Here's how the part is built. I have some questions about the finished solid (model axes, mm). Face numbers are marked on the shaded views. A direction names the side the tool comes from. Coordinates: 2 decimals unless noted, no trailing zeros. Loops run counter-clockwise (first coordinate to the right, second up) from the corner with the lowest first, then second, coordinate; pieces in that order, holes last. Notation, with made-up numbers: (-30.75, 3.5) -> (-1.75, 3.5) arc R12 cw to (-1.75, 17.5) -> close; hole circle Ø7 at (-16.5, 40.5). An arc over 180 degrees is marked (long way). Answer as a JSON object with one key per item and string values. Group by question number.
1) Which directions (+Z, -Z, +X, -X, +Y, -Y) give clear straight access to the entire face, cutting with the end or side of a thin tool? Please do the marked faces 1, 2, 3, 4 and 5.
2) I want a section at D-D (x = 11.5). Write out the boundary of the cut face in (y, z).
3) I want a section at A-A (y = 0). Write out the boundary of the cut face in (x, z) (3 decimals).
4) I want a section at C-C (x = 0). Count the separate pieces of the cut face and the enclosed holes in it, then the cut area to 3 significant figures.
5) If we mould it in two halves opening along X, with no side actions, what happens to the marked faces 6, 7, 8 and 9? For each: +X half, -X half, draft (parallel to the pull), parting line (faces both ways), or undercut.
6) I need wall thicknesses on probe 1 along Y at (x, z) = (0, 10) (3 decimals); probe 2 along Y at (x, z) = (0, 12); probe 3 along Z at (x, y) = (5, 19.5). Which ranges of each line are inside material? Lowest first, please. Write a range as [from, to].
7) I'm going to push flat-ended pins straight in: pin 1 (14 mm diameter, centred on x = -4, y = -5.5, fed in from -Z); pin 2 (3.5 mm diameter, centred on x = 0, z = 14, fed in from +Y); pin 3 (3 mm diameter, centred on y = 2, z = 5, fed in from -X); pin 4 (3 mm diameter, centred on x = -12.5, y = 12, fed in from -Z). Where does each tip first touch, or does it pass through?
8) I want a section at B-B (z = 6.75). Write out the boundary of the cut face in (x, y), then the cut area to 4 significant figures.
```python
from build123d import *
from build123d.topology import SkipClean

# Parameters (mm, degrees)
SKETCH2_R           = 14
SKETCH2_R_2         = 3.5
BOSS_EXTRUDE1_DEPTH = 5.5
SKETCH3_R           = 7
CUT_EXTRUDE1_DEPTH  = 39.255719
TAP1_REACH          = 49.937
TAP1_BORE_R         = 1.3105
CIRPATTERN1_COUNT   = 2
CIRPATTERN1_ANGLE   = 120


with BuildPart() as part:
    # Sketch1 → Revolve1 (revolve)
    with BuildSketch(Plane(origin=(0, 0, 0), x_dir=(0, 0, -1), z_dir=(1, 0, 0)), mode=Mode.PRIVATE) as revolve1_sk:
        with BuildLine():
            Line((-11.5, 19), (0, 19))
            Line((0, 19), (0, 14))
            Line((0, 14), (-1.5, 14))
            Line((-1.5, 14), (-1.5, 8.425))
            ThreePointArc((-1.5, 8.425), (-1.55, 8.375), (-1.5, 8.325))
            Line((-1.5, 8.325), (-1.5, 6))
            Line((-1.5, 6), (-16, 6))
            Line((-16, 6), (-16, 9.5))
            Line((-16, 9.5), (-11.5, 9.5))
            Line((-11.5, 9.5), (-11.5, 8.375))
            Line((-11.5, 8.375), (-9.5, 8.375))
            Line((-9.5, 8.375), (-9.5, 14))
            Line((-9.5, 14), (-11.5, 14))
            Line((-11.5, 14), (-11.5, 19))
        make_face()
    revolve(revolve1_sk.sketch.rotate(Axis((0, 0, 16), (0, 0, -1)), 90), axis=Axis((0, 0, 16), (0, 0, -1)))

    # Sketch2 → Boss-Extrude1 (add)
    with SkipClean():  # the faces are left unmerged after this step: merging them gives an invalid solid
        with BuildSketch(Plane.XY):
            with BuildLine():
                Line((-5.76484, 29.278248), (-12.6665, 14.161913))
                ThreePointArc((-12.6665, 14.161913), (-19, 0), (-12.6665, -14.161913))
                Line((-12.6665, -14.161913), (-5.76484, -29.278248))
                ThreePointArc((-5.76484, -29.278248), (-4.850203, -30.524474), (-3.514877, -31.303285))
                ThreePointArc((-3.514877, -31.303285), (0, -31.5), (3.514877, -31.303285))
                ThreePointArc((3.514877, -31.303285), (4.850203, -30.524474), (5.76484, -29.278248))
                Line((5.76484, -29.278248), (12.6665, -14.161913))
                ThreePointArc((12.6665, -14.161913), (19, 0), (12.6665, 14.161913))
                Line((12.6665, 14.161913), (5.76484, 29.278248))
                ThreePointArc((5.76484, 29.278248), (4.850203, 30.524474), (3.514877, 31.303285))
                ThreePointArc((3.514877, 31.303285), (0, 31.5), (-3.514877, 31.303285))
                ThreePointArc((-3.514877, 31.303285), (-4.850203, 30.524474), (-5.76484, 29.278248))
            make_face()
            Circle(SKETCH2_R, mode=Mode.SUBTRACT)
            with Locations((0, 24)):
                Circle(SKETCH2_R_2, mode=Mode.SUBTRACT)
            with Locations((0, -24)):
                Circle(SKETCH2_R_2, mode=Mode.SUBTRACT)
        extrude(amount=BOSS_EXTRUDE1_DEPTH)

    # Sketch3 → Cut-Extrude1 (cut, through all)
    with SkipClean():  # the faces are left unmerged after this step: merging them gives an invalid solid
        with BuildSketch(Plane.XY.offset(5.5)):
            with Locations((0, 24)):
                Circle(SKETCH3_R)
            with Locations((0, -24)):
                Circle(SKETCH3_R)
        extrude(amount=CUT_EXTRUDE1_DEPTH, mode=Mode.SUBTRACT)

    # Tap1 bore → Tap1 (cut, up to next)
    with BuildSketch(Plane(origin=(0, 9.5, 0), x_dir=(1, 0, 0), z_dir=(0, 1, 0)), mode=Mode.PRIVATE) as tap1_sk1:
        with Locations((0, -14)):
            Circle(TAP1_BORE_R)
    tap1_tool1 = extrude(tap1_sk1.sketch, amount=-TAP1_REACH, mode=Mode.PRIVATE) & part.part
    tap1 = tap1_tool1.solids().sort_by_distance((0, 9.5, 14))[0]
    add(tap1, mode=Mode.SUBTRACT)

    # CirPattern1: Tap1 ×2 about axis
    with SkipClean():  # the faces are left unmerged after this step: merging them gives an invalid solid
        cirpattern1_axis = Axis((0, 0, 16), (0, 0, 1))
        for i in range(1, CIRPATTERN1_COUNT):
            add(tap1.rotate(cirpattern1_axis, i * CIRPATTERN1_ANGLE / (CIRPATTERN1_COUNT - 1)), mode=Mode.SUBTRACT)


solid = part.part
```
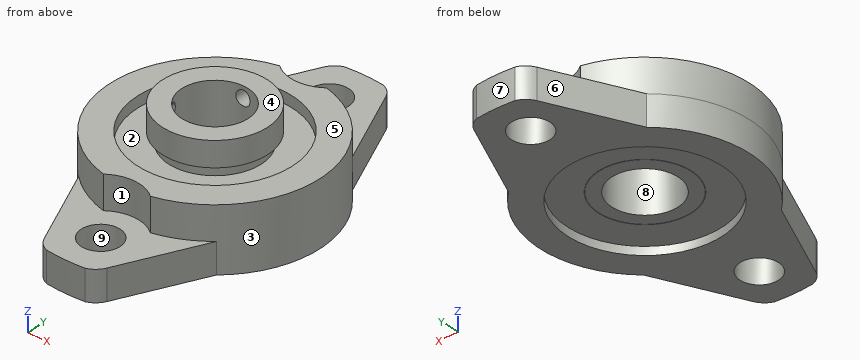
Determined:
{
 "1": {"face 1": "+Z, -Y", "face 2": "none", "face 3": "+Z, +X", "face 4": "+Z, +X, -X, +Y, -Y", "face 5": "+Z"},
 "2": {"outline": "(-16.72, 0) -> (-7.98, 0) -> (-7.98, 1.5) -> (7.98, 1.5) -> (7.98, 0) -> (16.72, 0) -> (16.72, 5.5) -> (15.12, 5.5) -> (15.12, 11.5) -> (7.98, 11.5) -> (7.98, 9.5) -> (-7.98, 9.5) -> (-7.98, 11.5) -> (-15.12, 11.5) -> (-15.12, 5.5) -> (-16.72, 5.5) -> close"},
 "3": {"outline": "(-19, 0) -> (-14, 0) -> (-14, 1.5) -> (-8.425, 1.5) arc R0.05 cw to (-8.325, 1.5) -> (-6, 1.5) -> (-6, 16) -> (-9.5, 16) -> (-9.5, 11.5) -> (-8.375, 11.5) -> (-8.375, 9.5) -> (-14, 9.5) -> (-14, 11.5) -> (-19, 11.5) -> close; (6, 1.5) -> (8.325, 1.5) arc R0.05 cw to (8.425, 1.5) -> (14, 1.5) -> (14, 0) -> (19, 0) -> (19, 11.5) -> (14, 11.5) -> (14, 9.5) -> (8.375, 9.5) -> (8.375, 11.5) -> (9.5, 11.5) -> (9.5, 16) -> (6, 16) -> close"},
 "4": {"separate pieces": "5", "enclosed holes": "0", "area": "311 mm^2"},
 "5": {"face 6": "-X half", "face 7": "parting line", "face 8": "undercut", "face 9": "undercut"},
 "6": {"probe 1": "[-17, -14], [-8.375, -6], [6, 8.375], [14, 17]", "probe 2": "[-9.5, -6], [6, 9.5]", "probe 3": "[0, 5.5]"},
 "7": {"pin 1": "z = 1.5", "pin 2": "y = 9.5", "pin 3": "x = -18.99", "pin 4": "z = 0"},
 "8": {"outline": "(-4.33, -18.5) arc R7 cw to (4.33, -18.5) arc R19 ccw to (4.33, 18.5) arc R7 cw to (-4.33, 18.5) arc R19 ccw to start; hole circle Ø12 at (0, 0)", "area": "997.5 mm^2"}
}
